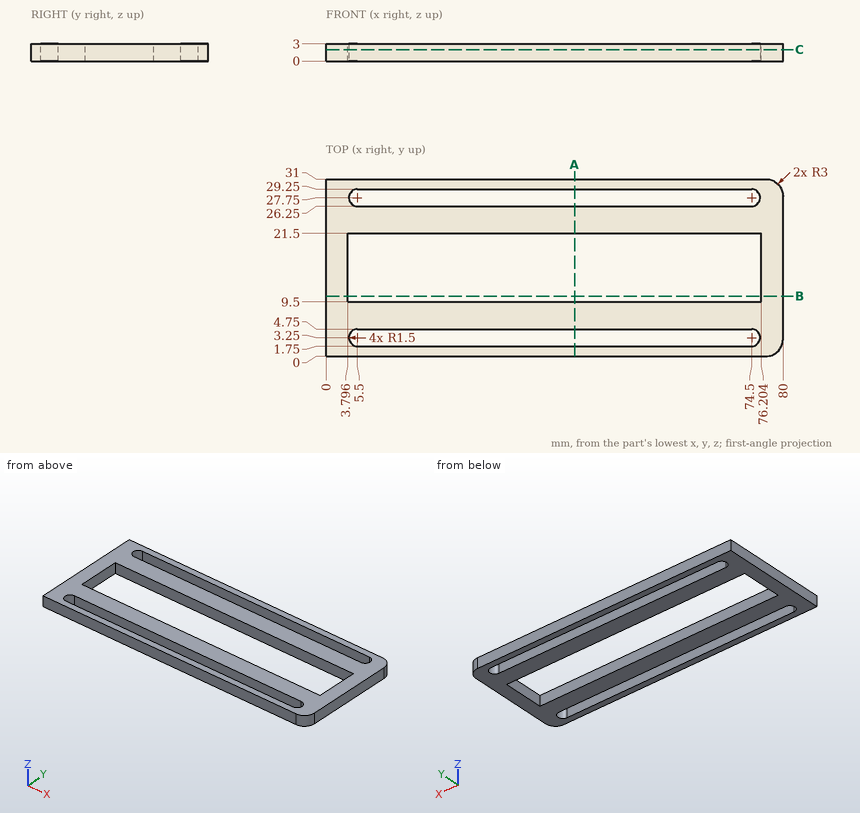
Verification items for this drawing (mm, ordinates from the low corner). Give positions to 0.01 mm unless a question says otherwise; leave off trailing zeros. Loops run counter-clockwise (first coordinate to the right, second up) from the corner with the lowest first, then second, coordinate; pieces in that order, holes last. Notation, with made-up numbers: M 85,-38.75 L 110,-38.75 A22 cw 110,-7.75 Z; hole C -39,5 d3. An arc over 180 degrees is marked long. Write each question's results on one line, items separated by ' | '.
1) Thickness scan on line 1 (Y direction, x = 57, z = 1.9); line 2 (X direction, y = 16, z = 0.7). Record the ranges inside material, lowest first.
Answers follow:
line 1: 0 to 1.75, 4.75 to 9.5, 21.5 to 26.25, 29.25 to 31 | line 2: 0 to 3.8, 76.2 to 80
2) Section check C-C, the plane z = 2. Record the boundary of the cut face in (x, y), plus the area to 3 significant figures.
Answers follow:
outline: M 0,0 L 77,0 A3 ccw 80,3 L 80,28 A3 ccw 77,31 L 0,31 Z; hole M 3.8,9.5 L 76.2,9.5 L 76.2,21.5 L 3.8,21.5 Z; hole M 5.5,1.75 L 74.5,1.75 A1.5 ccw 74.5,4.75 L 5.5,4.75 A1.5 ccw Z; hole M 5.5,26.25 L 74.5,26.25 A1.5 ccw 74.5,29.25 L 5.5,29.25 A1.5 ccw Z | area: 1,180 mm2
3) Section check A-A, the plane x = 43.5. Record the boundary of the cut face in (y, z), plus the area to 3 significant figures.
Answers follow:
outline: M 0,0 L 1.75,0 L 1.75,3 L 0,3 Z; M 4.75,0 L 9.5,0 L 9.5,3 L 4.75,3 Z; M 21.5,0 L 26.25,0 L 26.25,3 L 21.5,3 Z; M 29.25,0 L 31,0 L 31,3 L 29.25,3 Z | area: 39.0 mm2
4) Section check B-B, the plane y = 10.5. Record the boundary of the cut face in (x, z), plus the area to 3 significant figures.
Answers follow:
outline: M 0,0 L 3.8,0 L 3.8,3 L 0,3 Z; M 76.2,0 L 80,0 L 80,3 L 76.2,3 Z | area: 22.8 mm2
